```python
from build123d import *

# Parameters (mm, degrees)
SKETCH1_W                      = 40
SKETCH1_H                      = 22
BASE_FLANGE2_DEPTH             = 0.7366
EDGE_FLANGE2_STRIP_W           = 4.4196
EDGE_FLANGE2_STRIP_H           = 0.7366
EDGE_FLANGE2_STRIP_CUT_DEPTH   = 22
EDGE_FLANGE2_STRIP_2_W         = 4.4196
EDGE_FLANGE2_STRIP_2_H         = 0.7366
EDGE_FLANGE2_STRIP_CUT_2_DEPTH = 22
EDGE_FLANGE2_DEPTH             = 22
EDGE_FLANGE2_PROFILE_W         = 110
EDGE_FLANGE2_PROFILE_H         = 18.5268
EDGE_FLANGE2_FLAT_DEPTH        = 0.7366
EDGE_FLANGE2_BEND_DEPTH        = 22
EDGE_FLANGE2_PROFILE_2_W       = 110
EDGE_FLANGE2_PROFILE_2_H       = 18.5268
EDGE_FLANGE2_FLAT_2_DEPTH      = 0.7366
SKETCH32_R                     = 3.75
SKETCH32_R_2                   = 1.75
CUT_EXTRUDE1_DEPTH             = 2
CUT_EXTRUDE2_START             = -2
SKETCH33_R                     = 1.75
SKETCH33_R_2                   = 4
CUT_EXTRUDE2_DEPTH             = 2
CHAMFER1_SIZE                  = 2
CHAMFER2_SIZE                  = 10
SKETCH34_W                     = 23
SKETCH34_H                     = 12
CUT_EXTRUDE3_DEPTH             = 2


# Sheet-metal steps are written as plain solids
with BuildPart() as part:
    # Sketch1 → Base-Flange2 (new body)
    with BuildSketch(Plane(origin=(0, 0, 0), x_dir=(1, 0, 0), z_dir=(0, 1, 0))):
        Rectangle(SKETCH1_W, SKETCH1_H)
    extrude(amount=BASE_FLANGE2_DEPTH)

    # Edge-Flange2 strip (across the edge) → Edge-Flange2 strip cut (cut)
    with BuildSketch(Plane(origin=(20, 0, -11), x_dir=(-1, 0, 0), z_dir=(0, 0, 1))):
        with Locations((-0.7366, -0.3683)):
            Rectangle(EDGE_FLANGE2_STRIP_W, EDGE_FLANGE2_STRIP_H)
    extrude(amount=EDGE_FLANGE2_STRIP_CUT_DEPTH, mode=Mode.SUBTRACT)

    # Edge-Flange2 strip 2 (across the edge) → Edge-Flange2 strip cut 2 (cut)
    with BuildSketch(Plane(origin=(-20, 0, 11), x_dir=(1, 0, 0), z_dir=(0, 0, -1))):
        with Locations((-0.7366, -0.3683)):
            Rectangle(EDGE_FLANGE2_STRIP_2_W, EDGE_FLANGE2_STRIP_2_H)
    extrude(amount=EDGE_FLANGE2_STRIP_CUT_2_DEPTH, mode=Mode.SUBTRACT)

    # Edge-Flange2 bend section (across the edge) → Edge-Flange2 (add)
    with BuildSketch(Plane(origin=(20, 0, -11), x_dir=(-1, 0, 0), z_dir=(0, 0, 1))):
        with BuildLine():
            Line((0, 0.7366), (0.7366, 0.7366))
            ThreePointArc((0.7366, 0.7366), (0.952345145, 0.215745145), (1.4732, 0))
            Line((1.4732, 0), (1.4732, -0.7366))
            ThreePointArc((1.4732, -0.7366), (0.43149029, -0.30510971), (0, 0.7366))
        make_face()
    extrude(amount=EDGE_FLANGE2_DEPTH)

    # Edge-Flange2 profile (on flange) → Edge-Flange2 flat (add)
    with BuildSketch(Plane(origin=(20, 0, 0), x_dir=(0, 0, -1), z_dir=(-1, 0, 0))):
        with Locations((44, 10)):
            Rectangle(EDGE_FLANGE2_PROFILE_W, EDGE_FLANGE2_PROFILE_H)
    extrude(amount=EDGE_FLANGE2_FLAT_DEPTH)

    # Edge-Flange2 bend section 2 (across the edge) → Edge-Flange2 bend (add)
    with BuildSketch(Plane(origin=(-20, 0, 11), x_dir=(1, 0, 0), z_dir=(0, 0, -1))):
        with BuildLine():
            Line((0, 0.7366), (0.7366, 0.7366))
            ThreePointArc((0.7366, 0.7366), (0.952345145, 0.215745145), (1.4732, 0))
            Line((1.4732, 0), (1.4732, -0.7366))
            ThreePointArc((1.4732, -0.7366), (0.43149029, -0.30510971), (0, 0.7366))
        make_face()
    extrude(amount=EDGE_FLANGE2_BEND_DEPTH)

    # Edge-Flange2 profile 2 (on flange) → Edge-Flange2 flat 2 (add)
    with BuildSketch(Plane(origin=(-20, 0, 0), x_dir=(0, 0, 1), z_dir=(1, 0, 0))):
        with Locations((-44, 10)):
            Rectangle(EDGE_FLANGE2_PROFILE_2_W, EDGE_FLANGE2_PROFILE_2_H)
    extrude(amount=EDGE_FLANGE2_FLAT_2_DEPTH)

    # Sketch32 → Cut-Extrude1 (cut)
    with BuildSketch(Plane.ZY.offset(20)):
        with Locations(Location((-79, -10, 0), (0, 0, 270))):
            Circle(SKETCH32_R)
        with Locations(Location((-44, -10, 0), (0, 0, 270))):
            Circle(SKETCH32_R_2)
    extrude(amount=-CUT_EXTRUDE1_DEPTH, mode=Mode.SUBTRACT)

    # Sketch33 → Cut-Extrude2 (cut)
    with BuildSketch(Plane(origin=(20, 0, 0), x_dir=(0, 0, -1), z_dir=(1, 0, 0)).offset(CUT_EXTRUDE2_START)):
        with Locations(Location((44, -10, 0), (0, 0, 270))):
            Circle(SKETCH33_R)
        with Locations(Location((79, -10, 0), (0, 0, 90))):
            Circle(SKETCH33_R_2)
    extrude(amount=CUT_EXTRUDE2_DEPTH, mode=Mode.SUBTRACT)

    # Chamfer1
    chamfer1_edges = [part.edges().sort_by_distance(p)[0] for p in [
        (19.6317, -0.7366, -99),
        (19.6317, -19.2634, -99),
        (-19.6317, -0.7366, -99),
        (-19.6317, -19.2634, -99),
    ]]
    chamfer(chamfer1_edges, length=CHAMFER1_SIZE)

    # Chamfer2
    chamfer2_edges = [part.edges().sort_by_distance(p)[0] for p in [
        (19.6317, -19.2634, 11),
        (-19.6317, -19.2634, 11),
    ]]
    chamfer(chamfer2_edges, length=CHAMFER2_SIZE)

    # Sketch34 → Cut-Extrude3 (cut)
    with BuildSketch(Plane(origin=(0, 0.7366, 0), x_dir=(1, 0, 0), z_dir=(0, 1, 0))):
        Rectangle(SKETCH34_W, SKETCH34_H)
    extrude(amount=-CUT_EXTRUDE3_DEPTH, mode=Mode.SUBTRACT)


solid = part.part
```
For this review, take the finished solid that the model builds, in its own axes (mm). A direction names the side the tool comes from. Coordinates: 2 decimals unless noted, no trailing zeros. Write each loop counter-clockwise with the first axis right and the second up, starting at its lowest first coordinate (ties: lowest second). Pieces come first, ordered by that corner, then holes. Notation, with made-up numbers: (-21.75, 84.25) - (16.25, 84.25) arc R34 ccw to (16.25, 115.25) - close; hole circle Ø8 at (35, -32). An arc over 180 degrees is marked (long way). Answer in a Markdown table with one row per item. Add a question column.
Q1. For probe 1 along Y at (x, z) = (19.5, -79); probe 2 along X at (y, z) = (-14.5, -8.5); probe 3 along Z at (x, y) = (19.85, -10), list the stretches that pass through material, from the lowest coordinate up.
Q2. We need section C-C, the plane y = -4.25. State the section outline as (x, z) points, and give its area (3 significant figures).
Q3. We need section A-A, the plane z = -4. State the section outline as (x, y) points.
Q4. Draft analysis for pull direction Z (two halves, no side actions). For faces 1 (the cylindrical face through (-19.64, -9.62, -45.71)), 2 (the flat face through (0, 0, -7)), 3 (the flat face through (19.637, -18.249, -98.014)), state which applies: +Z half, -Z half, draft (parallel to the pull), parting line (faces both ways), or undercut.
Q5. We need section B-B, the plane x = -9.5. State the section outline as (y, z) points, and give its area (3 significant figures).
Q6. For P1, Ø0.6, axis at y = 0, z = 1, coming from the +X side; P2, Ø11, axis at x = -7, z = -4, coming from the -Y side; P3, Ø0.7, axis at x = -6, y = 0, coming from the -Z side, all flat-tipped, find the tip position at first contact; note any pin that passes through.
Q7. We need section D-D, the plane z = -44. State the section outline as (x, y) points.
Q8. Tool access review of faces 4 (the flat face through (-6, 0.2, 11)), 5 (the flat face through (-19.263, -8, -45)), 6 (the cylindrical face through (19.627, -10.867, -82.905)): name each direction out of +Z, -Z, +X, -X, +Y, -Y from which nothing blocks a thin tool from reaching the whole face with its end or side.
Answer list:
| question | item | result |
|---|---|---|
| 1 | probe 1 | y = -19.26 to -14, -6 to -0.74 |
| 1 | probe 2 | x = -20 to -19.26, 19.26 to 20 |
| 1 | probe 3 | z = -99 to -83, -75 to -45.75, -42.25 to 10.26 |
| 2 | outline | (-20, -99) - (-19.26, -99) - (-19.26, 11) - (-20, 11) - close; (19.26, -99) - (20, -99) - (20, 11) - (19.26, 11) - close |
| 2 | area | 162 mm2 |
| 3 | outline | (-20, -19.26) - (-19.26, -19.26) - (-19.26, -0.74) arc R0.74 cw to (-18.53, 0) - (-11.5, 0) - (-11.5, 0.74) - (-18.53, 0.74) arc R1.47 ccw to (-20, -0.74) - close; (11.5, 0) - (18.53, 0) arc R0.74 cw to (19.26, -0.74) - (19.26, -19.26) - (20, -19.26) - (20, -0.74) arc R1.47 ccw to (18.53, 0.74) - (11.5, 0.74) - close |
| 4 | face 1 | undercut |
| 4 | face 2 | draft |
| 4 | face 3 | -Z half |
| 5 | outline | (0, -11) - (0.74, -11) - (0.74, -6) - (0, -6) - close; (0, 6) - (0.74, 6) - (0.74, 11) - (0, 11) - close |
| 5 | area | 7.37 mm2 |
| 6 | P1 | stops at x = 19.93 |
| 6 | P2 | stops at y = 0 |
| 6 | P3 | stops at z = -11 |
| 7 | outline | (-20, -19.26) - (-19.26, -19.26) - (-19.26, -11.75) - (-20, -11.75) - close; (-20, -8.25) - (-19.26, -8.25) - (-19.26, -0.74) - (-20, -0.74) - close; (19.26, -19.26) - (20, -19.26) - (20, -11.75) - (19.26, -11.75) - close; (19.26, -8.25) - (20, -8.25) - (20, -0.74) - (19.26, -0.74) - close |
| 8 | face 4 | +Z, +X, -X, +Y, -Y |
| 8 | face 5 | +Z, -Z, -Y |
| 8 | face 6 | +X |
